```python
from build123d import *

# Parameters (mm, degrees)
SKETCH1_W           = 130
SKETCH1_H           = 114.8
SKETCH1_R           = 1.55
BOSS_EXTRUDE1_DEPTH = 3
CUT_EXTRUDE1_REACH  = 5
SKETCH3_R           = 1.55
CUT_EXTRUDE2_REACH  = 5
SKETCH4_R           = 1.55


with BuildPart() as part:
    # Sketch1 → Boss-Extrude1 (new body)
    with BuildSketch(Plane.XY):
        Rectangle(SKETCH1_W, SKETCH1_H)
        with Locations((-59.5, 44.4)):
            Circle(SKETCH1_R, mode=Mode.SUBTRACT)
        with Locations((58, 44.4)):
            Circle(SKETCH1_R, mode=Mode.SUBTRACT)
        with Locations((58, -47.4)):
            Circle(SKETCH1_R, mode=Mode.SUBTRACT)
        with Locations((-59.5, -47.4)):
            Circle(SKETCH1_R, mode=Mode.SUBTRACT)
    extrude(amount=BOSS_EXTRUDE1_DEPTH)

    # Sketch3 → Cut-Extrude1 (cut, up to next)
    with BuildSketch(Plane(origin=(0, 0, 0), x_dir=(-1, 0, 0), z_dir=(0, 0, -1)), mode=Mode.PRIVATE) as cut_extrude1_sk1:
        with Locations((-50, -29.4)):
            Circle(SKETCH3_R)
    cut_extrude1_tool1 = extrude(cut_extrude1_sk1.sketch, amount=-CUT_EXTRUDE1_REACH, mode=Mode.PRIVATE) & part.part
    add(cut_extrude1_tool1.solids().sort_by_distance((50, -29.4, 0))[0], mode=Mode.SUBTRACT)
    # Sketch3 → Cut-Extrude1 (cut, up to next)
    with BuildSketch(Plane(origin=(0, 0, 0), x_dir=(-1, 0, 0), z_dir=(0, 0, -1)), mode=Mode.PRIVATE) as cut_extrude1_sk2:
        with Locations((50, -29.4)):
            Circle(SKETCH3_R)
    cut_extrude1_tool2 = extrude(cut_extrude1_sk2.sketch, amount=-CUT_EXTRUDE1_REACH, mode=Mode.PRIVATE) & part.part
    add(cut_extrude1_tool2.solids().sort_by_distance((-50, -29.4, 0))[0], mode=Mode.SUBTRACT)

    # Sketch4 → Cut-Extrude2 (cut, up to next)
    with BuildSketch(Plane(origin=(0, 0, 0), x_dir=(-1, 0, 0), z_dir=(0, 0, -1)), mode=Mode.PRIVATE) as cut_extrude2_sk1:
        with Locations((-34.6, 44.4)):
            Circle(SKETCH4_R)
    cut_extrude2_tool1 = extrude(cut_extrude2_sk1.sketch, amount=-CUT_EXTRUDE2_REACH, mode=Mode.PRIVATE) & part.part
    add(cut_extrude2_tool1.solids().sort_by_distance((34.6, 44.4, 0))[0], mode=Mode.SUBTRACT)
    # Sketch4 → Cut-Extrude2 (cut, up to next)
    with BuildSketch(Plane(origin=(0, 0, 0), x_dir=(-1, 0, 0), z_dir=(0, 0, -1)), mode=Mode.PRIVATE) as cut_extrude2_sk2:
        with Locations((17.4, 25.96)):
            Circle(SKETCH4_R)
    cut_extrude2_tool2 = extrude(cut_extrude2_sk2.sketch, amount=-CUT_EXTRUDE2_REACH, mode=Mode.PRIVATE) & part.part
    add(cut_extrude2_tool2.solids().sort_by_distance((-17.4, 25.96, 0))[0], mode=Mode.SUBTRACT)


solid = part.part
```
CAD build for the part. Positions are in the model's coordinates, mm. Coordinates: 2 decimals unless noted, no trailing zeros. Order: outer loops, then holes, each group sorted by start corner. A loop starts at its lowest first (then second) coordinate and runs counter-clockwise, first axis right, second up.
(1) Saw through at D-D, the plane y = 44.4. Write the cut outline in (x, z).
Solution:
outline: (-65, 0) - (-61.05, 0) - (-61.05, 3) - (-65, 3) - close; (-57.95, 0) - (33.05, 0) - (33.05, 3) - (-57.95, 3) - close; (36.15, 0) - (56.45, 0) - (56.45, 3) - (36.15, 3) - close; (59.55, 0) - (65, 0) - (65, 3) - (59.55, 3) - close
(2) Mould opens along X. For faces 1 (the face through (-1, 1, 0)), 2 (the face through (-65, -1, 1)), 3 (the face through (48.522, -28.934, 1.479)) say: released by +X, released by -X, zero draft, split by the parting line, or undercut.
Solution:
face 1: zero draft
face 2: released by -X
face 3: undercut
(3) Saw through at A-A, the plane x = -59.5. Write the cut outline in (y, z), and give its area (3 significant figures).
Solution:
outline: (-57.4, 0) - (-48.95, 0) - (-48.95, 3) - (-57.4, 3) - close; (-45.85, 0) - (42.85, 0) - (42.85, 3) - (-45.85, 3) - close; (45.95, 0) - (57.4, 0) - (57.4, 3) - (45.95, 3) - close
area: 326 mm2
(4) Drill centre lines: L1, parallel to Y at x = -59.5, z = 2.25; L2, parallel to X at y = -48, z = 2.85; L3, parallel to Y at x = -50, z = 1.7. Where is each one in solid material? Low to high.
Solution:
L1: y = -57.4 to -48.95, -45.85 to 42.85, 45.95 to 57.4
L2: x = -65 to -60.93, -58.07 to 56.57, 59.43 to 65
L3: y = -57.4 to -30.95, -27.85 to 57.4
(5) Pin check, flat tip, straight feed: pin 1 Ø1.9 at (x, y) = (-59.5, -47.4) entering from +Z. Stop position of the tip, or through.
Solution:
pin 1: passes through
(6) Saw through at C-C, the plane y = 25.96. Write the cut outline in (x, z), and give its area (3 significant figures).
Solution:
outline: (-65, 0) - (-18.95, 0) - (-18.95, 3) - (-65, 3) - close; (-15.85, 0) - (65, 0) - (65, 3) - (-15.85, 3) - close
area: 381 mm2
(7) Saw through at B-B, the plane y = -29.4. Write the cut outline in (x, z).
Solution:
outline: (-65, 0) - (-51.55, 0) - (-51.55, 3) - (-65, 3) - close; (-48.45, 0) - (48.45, 0) - (48.45, 3) - (-48.45, 3) - close; (51.55, 0) - (65, 0) - (65, 3) - (51.55, 3) - close
